```python
from build123d import *

# Parameters (mm, degrees)
SKETCH1_R           = 4.05
BOSS_EXTRUDE1_DEPTH = 5
SCALE1_SCALE        = 0.471698113
SKETCH2_R           = 1.910377358
BOSS_EXTRUDE2_DEPTH = 4.716981
SKETCH3_R           = 9.5
CUT_EXTRUDE1_DEPTH  = 78.491048109
FILLET1_R           = 20


with BuildPart() as part:
    # Sketch1 → Boss-Extrude1 (new, symmetric)
    with BuildSketch(Plane(origin=(0, 0, 0), x_dir=(1, 0, 0), z_dir=(0, 1, 0))):
        with BuildLine():
            Line((-115.945353012, 22.704926206), (-2.044938074, -7.668517777))
            ThreePointArc((-2.044938074, -7.668517777), (-0.023122965, -7.936460291), (2.000219114, -7.680303388))
            Line((2.000219114, -7.680303388), (116.075928336, 22.028993564))
            ThreePointArc((116.075928336, 22.028993564), (121.992194313, 31.992800071), (112.09054435, 38.012515284))
            ThreePointArc((112.09054435, 38.012515284), (-0.062996347, 24.666684437), (-112.292885137, 37.35447203))
            ThreePointArc((-112.292885137, 37.35447203), (-121.325741435, 31.826475412), (-115.945353012, 22.704926206))
        make_face()
        with Locations(Location((0, 0, 0), (0, 0, 270))):
            Circle(SKETCH1_R, mode=Mode.SUBTRACT)
        with Locations(Location((114, 30, 0), (0, 0, 270))):
            Circle(SKETCH1_R, mode=Mode.SUBTRACT)
        with Locations(Location((-114, 30, 0), (0, 0, 270))):
            Circle(SKETCH1_R, mode=Mode.SUBTRACT)
    extrude(amount=BOSS_EXTRUDE1_DEPTH, both=True)


with BuildPart() as part_1:
    # Scale1: scaled about (1.578802129, 0, -17.052920202)
    add(part.part.scale(SCALE1_SCALE).moved(Location((0.834084144, 0, -9.009089918))))

    # Sketch2 → Boss-Extrude2 (add, through all)
    with BuildSketch(Plane(origin=(0, 2.358490566, 0), x_dir=(1, 0, 0), z_dir=(0, 1, 0))):
        with BuildLine():
            Line((13.487042299, 4.302429752), (45.990989369, 12.76759225))
            ThreePointArc((45.990989369, 12.76759225), (67.744107555, 26.27194324), (42.244562907, 28.582542559))
            ThreePointArc((42.244562907, 28.582542559), (0.907570824, 24.644667364), (-40.455525682, 28.298161983))
            ThreePointArc((-40.455525682, 28.298161983), (-66.076792027, 26.268341249), (-44.081633602, 12.97238445))
            Line((-44.081633602, 12.97238445), (-11.846084783, 4.376238098))
            ThreePointArc((-11.846084783, 4.376238098), (0.794751912, -4.490852784), (13.487042299, 4.302429752))
        make_face()
        with Locations(Location((54.607669049, 23.160033314, 0), (0, 0, 270))):
            Circle(SKETCH2_R, mode=Mode.SUBTRACT)
        with Locations(Location((0.834084144, 9.009089918, 0), (0, 0, 270))):
            Circle(SKETCH2_R, mode=Mode.SUBTRACT)
        with Locations(Location((-52.939500762, 23.160033314, 0), (0, 0, 270))):
            Circle(SKETCH2_R, mode=Mode.SUBTRACT)
    extrude(amount=-BOSS_EXTRUDE2_DEPTH)

    # Sketch3 → Cut-Extrude1 (cut, through all)
    with BuildSketch(Plane(origin=(0, 2.358490566, 0), x_dir=(1, 0, 0), z_dir=(0, 1, 0))):
        with Locations(Location((-52.939500762, 23.160033314, 0), (0, 0, 270))):
            Circle(SKETCH3_R)
        with Locations(Location((0.834084144, 9.009089918, 0), (0, 0, 270))):
            Circle(SKETCH3_R)
        with Locations(Location((54.607669049, 23.160033314, 0), (0, 0, 270))):
            Circle(SKETCH3_R)
    extrude(amount=-CUT_EXTRUDE1_DEPTH, mode=Mode.SUBTRACT)

    # Fillet1
    fillet1_edges = [part_1.edges().sort_by_distance(p)[0] for p in [
        (42.244562907, 6.6e-08, -28.582542559),
        (45.990989369, 6.6e-08, -12.76759225),
        (13.487042299, 6.6e-08, -4.302429752),
        (-11.846084783, 6.6e-08, -4.376238098),
        (-44.081633602, 6.6e-08, -12.97238445),
        (-40.455525682, 6.6e-08, -28.298161983),
    ]]
    fillet(fillet1_edges, radius=FILLET1_R)


solid = part_1.part
```
Design review of the part built by this model. Coordinates are the model's own, in mm. A direction names the side the tool comes from. Give positions to 0.01 mm unless a question says otherwise; leave off trailing zeros. Order: outer loops, then holes, each group sorted by start corner. A loop starts at its lowest first (then second) coordinate and runs counter-clockwise, first axis right, second up. Notation, with made-up numbers: (71.25, 20.25) - (94.25, 20.25) arc R32 ccw to (94.25, 49.25) - close; hole circle Ø7 at (60, -36.5). An arc over 180 degrees is marked (long way). Use a Markdown table: item, result. Add a question column.
(1) Machinability: for faces 1 (the face through (29.669, 0.033, -8.517)), 2 (the face through (-62.214, 0.033, -25.219)), which of the approach directions +Z, -Z, +X, -X, +Y, -Y give a long, thin tool a straight path to every point of the face, cutting with its end or side? Answer none if there is none.
(2) Add section C-C on z = -4. Give the boundary of the cut face in (x, y).
(3) Wall thickness on probe 1 along Z at (x, y) = (1, 0.15) (3 decimals); probe 2 along X at (y, z) = (-1, -14.5); probe 3 along X at (y, z) = (-0.6, -19): over which ranges is each line inside the solid? List them lowest first. Write a range as [from, to].
(4) Add section A-A on z = -21.5. Give the boundary of the cut face in (x, y), then the cut area to 3 significant figures.
(5) Mouldability with a two-part tool opening along X and no side actions: class faces 3 (the face through (-42.39, -0.03, -11.61)), 4 (the face through (15.575, -0.033, -3.964)), 5 (the face through (0, 2.358, -21)) as +X half, -X half, draft (parallel to the pull), parting line (faces both ways), or undercut.
(6) Add section B-B on x = -7. Give the boundary of the cut face in (y, z), then the cut area to 3 significant figures.
(7) Clearance check with flat-ended pins moving along their axes: P1, Ø2, axis at y = 1.5, z = -26, coming from the +X side; P2, Ø1.5, axis at x = -34.5, y = -2, coming from the +Z side; P3, Ø17, axis at x = -52.94, z = -23.16, coming from the +Y side; P4, Ø1.5, axis at x = -25.5, y = -1.5, coming from the -Z side. State where each tip first meets the part, or that it passes through.
(8) Add section D-D on x = 59.5. Give the boundary of the cut face in (y, z), then the cut area to 3 significant figures.
Report:
| question | item | result |
|---|---|---|
| 1 | face 1 | +Z, +Y, -Y |
| 1 | face 2 | +Y, -Y |
| 2 | outline | (-13.86, -2.36) - (-7.24, -2.36) - (-7.24, 2.36) - (-13.86, 2.36) - close; (8.91, -2.36) - (15.64, -2.36) - (15.64, 2.36) - (8.91, 2.36) - close |
| 3 | probe 1 | z = [-24.645, -18.508], [0.489, 4.49] |
| 3 | probe 2 | x = [-63.3, -56.85], [-49.03, -6.92], [8.59, 50.7], [58.51, 64.96] |
| 3 | probe 3 | x = [-65.78, -61.48], [-44.4, 46.07], [63.15, 67.45] |
| 4 | outline | (-66.34, -2.36) - (-62.29, -2.36) - (-62.29, 2.36) - (-66.34, 2.36) - close; (-43.59, -2.36) - (45.25, -2.36) - (45.25, 2.36) - (-43.59, 2.36) - close; (63.96, -2.36) - (68.01, -2.36) - (68.01, 2.36) - (63.96, 2.36) - close |
| 4 | area | 457 mm² |
| 5 | face 3 | undercut |
| 5 | face 4 | +X half |
| 5 | face 5 | draft |
| 6 | outline | (-2.36, -24.76) - (2.36, -24.76) - (2.36, -14.38) - (-2.36, -14.38) - close; (-2.36, -3.64) - (2.36, -3.64) - (2.36, 1.99) - (-2.36, 1.99) - close |
| 6 | area | 75.4 mm² |
| 7 | P1 | stops at x = 67.98 |
| 7 | P2 | stops at z = -10.22 |
| 7 | P3 | passes through |
| 7 | P4 | stops at z = -26.18 |
| 8 | outline | (-2.36, -35.74) - (2.36, -35.74) - (2.36, -31.3) - (-2.36, -31.3) - close; (-2.36, -15.02) - (2.36, -15.02) - (2.36, -10.58) - (-2.36, -10.58) - close |
| 8 | area | 41.9 mm² |
